Input: part model. Units: mm. Frame: model coordinates. Face numbers are marked on the shaded views. Round coordinates to 2 decimals unless told otherwise and drop trailing zeros. Loops run counter-clockwise (first coordinate to the right, second up) from the corner with the lowest first, then second, coordinate; pieces in that order, holes last. Notation, with made-up numbers: M 44,89.25 L 98,89.25 A21 cw 98,108.25 Z; hole C -38.75,-25 d8. An arc over 180 degrees is marked long. Put each result on its own line as item: value. Start each with the question number.
1) Draft query along Z for the marked faces 1 and 2. Return one class per face: +Z half, -Z half, draft (parallel to the pull), parting line (faces both ways), or undercut.
2) Line query: probe 1 along X at (y, z) = (-1.25, 0); probe 2 along Z at (x, y) = (21.5, -1.25); probe 3 along X at (y, z) = (0.15, 2). Output: solid intervals per line, ascending.
3) Section C-C on y = 0.1. Output: boundary loops of the cut face in (x, z).
4) Section B-B on z = 0. Output: boundary loops of the cut face in (x, y), plus the area to 3 significant figures.
5) Section A-A on x = -21.5. Output: boundary loops of the cut face in (y, z).
6) Pin query (flat end, axial travel): pin 1 (5.5 mm diameter, centred on x = 21.5, z = 0, fed in from +Y). Return the tip coordinate at first contact, or that it passes through.
from build123d import *

# Parameters (mm, degrees)
EXTRUDE_765_DEPTH           = 10
EXTRUDE_765_DEPTH_BACK      = 10
HOLE_WIZARD_M3_2_AT_2_COUNT = 2
HOLE_WIZARD_M3_2_AT_2_PITCH = 43


with BuildPart() as part:
    # Sketch 1 → Extrude 765 (new, two sides: drawn at the far end of the back side and taken through both)
    with BuildSketch(Plane.XY.offset(-EXTRUDE_765_DEPTH_BACK)):
        Polygon((29.5, 0.5), (-29.5, 0.5), (-29.5, -1.5), (-13.5, -1.5), (13.5, -1.5), (29.5, -1.5), align=None)
    extrude(amount=EXTRUDE_765_DEPTH + EXTRUDE_765_DEPTH_BACK)

    # Sketch 9 → Hole Wizard M3_2 (revolve, cut)
    with BuildSketch(Plane(origin=(-21.5, 0.5, 0), x_dir=(0, 0, 1), z_dir=(1, 0, 0))):
        Polygon((0, 0), (0, 2), (1.7, 2), (1.7, 1.66), (3.36, 0), align=None)
    hole_wizard_m3_2 = revolve(axis=Axis((-21.5, 6.85, 0), (0, -1, 0)), mode=Mode.SUBTRACT)

    # Hole Wizard M3_2 at 2: Hole Wizard M3_2 ×2
    with Locations(*[(i * HOLE_WIZARD_M3_2_AT_2_PITCH, 0, 0) for i in range(1, HOLE_WIZARD_M3_2_AT_2_COUNT)]):
        add(hole_wizard_m3_2, mode=Mode.SUBTRACT)


solid = part.part
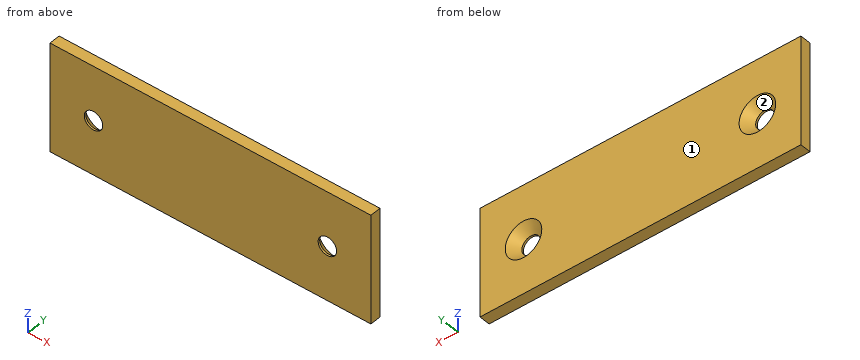
Geometry results:
1. face 1: draft
1. face 2: undercut
2. probe 1: x = -29.5 to -23.2, -19.8 to 19.8, 23.2 to 29.5
2. probe 2: z = -10 to -1.7, 1.7 to 10
2. probe 3: x = -29.5 to -23.75, -19.25 to 19.25, 23.75 to 29.5
3. outline: M -29.5,-10 L 29.5,-10 L 29.5,10 L -29.5,10 Z; hole C -21.5,0 d5.92; hole C 21.5,0 d5.92
4. outline: M -29.5,-1.5 L -23.2,-1.5 L -23.2,-1.16 L -24.86,0.5 L -29.5,0.5 Z; M -19.8,-1.5 L 19.8,-1.5 L 19.8,-1.16 L 18.14,0.5 L -18.14,0.5 L -19.8,-1.16 Z; M 23.2,-1.5 L 29.5,-1.5 L 29.5,0.5 L 24.86,0.5 L 23.2,-1.16 Z
4. area: 98.9 mm²
5. outline: M -1.5,-10 L 0.5,-10 L 0.5,-3.36 L -1.16,-1.7 L -1.5,-1.7 Z; M -1.5,1.7 L -1.16,1.7 L 0.5,3.36 L 0.5,10 L -1.5,10 Z
6. pin 1: stops at y = -0.11
